from build123d import *

# Parameters (mm, degrees)
TRAY_BLOCK_DEPTH              = 24.4
LOWER_FRONT_FACET_DEPTH       = 74.975401317
LOWER_FRONT_FACET_DEPTH_BACK  = 74.975401317
LOWER_SIDE_FACET_L_DEPTH      = 74.975401317
LOWER_SIDE_FACET_L_DEPTH_BACK = 74.975401317
LOWER_SIDE_FACET_R_DEPTH      = 74.975401317
LOWER_SIDE_FACET_R_DEPTH_BACK = 74.975401317
SHELL_T                       = -2.4
SEAM_REBATE_DEPTH             = 4.3
SKETCH6_R                     = 2.5
BOARD_PILLARS_DEPTH           = 24.9
SKETCH7_R                     = 0.8
BOARD_PILOTS_DEPTH            = 8.5
SKETCH8_W                     = 40
SKETCH8_H                     = 21
CABLE_WINDOW_DEPTH            = 3.9
SKETCH9_R                     = 4
FLANGE_BOSSES_DEPTH           = 6.2
SKETCH10_R                    = 2
FLANGE_INSERT_HOLES_DEPTH     = 7
SKETCH11_R                    = 1.7
SEAM_SCREW_HOLE_L_DEPTH       = 3.9
SKETCH12_R                    = 1.7
SEAM_SCREW_HOLE_R_DEPTH       = 3.9
SKETCH13_W                    = 12
SKETCH13_H                    = 7
BUNDLE_TIE_ANCHOR_DEPTH       = 5
SKETCH14_W                    = 4
SKETCH14_H                    = 2
BUNDLE_TIE_SLOT_DEPTH         = 14
SKETCH15_R                    = 1.5
DRAIN_HOLE_DEPTH              = 3.9


with BuildPart() as part:
    # Sketch1 → Tray Block (new body)
    with BuildSketch(Plane(origin=(0, -28.4, 0), x_dir=(1, 0, 0), z_dir=(0, 1, 0))):
        Polygon((-48.4, -11.9), (48.4, -11.9), (48.4, 42.2), (42.4, 48.2), (-42.4, 48.2), (-48.4, 42.2), align=None)
    extrude(amount=TRAY_BLOCK_DEPTH)

    # Sketch2 → Lower Front Facet (cut, two sides: drawn at the far end of the back side and taken through both)
    with BuildSketch(Plane(origin=(0, 0, 0), x_dir=(0, 0, -1), z_dir=(1, 0, 0)).offset(-LOWER_FRONT_FACET_DEPTH_BACK)):
        Polygon((49.64, -6.32), (53.2, -6.32), (53.2, -32.08), (39.56, -32.08), align=None)
    extrude(amount=LOWER_FRONT_FACET_DEPTH + LOWER_FRONT_FACET_DEPTH_BACK, mode=Mode.SUBTRACT)

    # Sketch3 → Lower Side Facet L (cut, two sides: drawn at the far end of the back side and taken through both)
    with BuildSketch(Plane.XY.offset(-LOWER_SIDE_FACET_L_DEPTH_BACK)):
        Polygon((-49.4, -21.4), (-49.4, -29.4), (-41.4, -29.4), align=None)
    extrude(amount=LOWER_SIDE_FACET_L_DEPTH + LOWER_SIDE_FACET_L_DEPTH_BACK, mode=Mode.SUBTRACT)

    # Sketch4 → Lower Side Facet R (cut, two sides: drawn at the far end of the back side and taken through both)
    with BuildSketch(Plane.XY.offset(-LOWER_SIDE_FACET_R_DEPTH_BACK)):
        Polygon((49.4, -21.4), (49.4, -29.4), (41.4, -29.4), align=None)
    extrude(amount=LOWER_SIDE_FACET_R_DEPTH + LOWER_SIDE_FACET_R_DEPTH_BACK, mode=Mode.SUBTRACT)

    # Shell
    shell_openings = [part.faces().sort_by_distance(p)[0] for p in [
        (0, -4, -17.975344882),
    ]]
    offset(amount=SHELL_T, openings=shell_openings, kind=Kind.INTERSECTION)

    # Sketch5 → Seam Rebate (cut)
    with BuildSketch(Plane(origin=(0, -7.3, 0), x_dir=(1, 0, 0), z_dir=(0, 1, 0))):
        Polygon((-46.3, -9.8), (46.3, -9.8), (46.3, 41.330151519), (41.530151519, 46.1), (-41.530151519, 46.1), (-46.3, 41.330151519), align=None)
    extrude(amount=SEAM_REBATE_DEPTH, mode=Mode.SUBTRACT)

    # Sketch6 → Board Pillars (add)
    with BuildSketch(Plane(origin=(0, -26.5, 0), x_dir=(1, 0, 0), z_dir=(0, 1, 0))):
        with Locations(Location((-11.3, 11.8, 0), (0, 0, 270))):
            Circle(SKETCH6_R)
        with Locations(Location((-11.3, 34.9, 0), (0, 0, 270))):
            Circle(SKETCH6_R)
        with Locations(Location((11.3, 11.8, 0), (0, 0, 270))):
            Circle(SKETCH6_R)
        with Locations(Location((11.3, 34.9, 0), (0, 0, 270))):
            Circle(SKETCH6_R)
    extrude(amount=BOARD_PILLARS_DEPTH)

    # Sketch7 → Board Pilots (cut)
    with BuildSketch(Plane(origin=(0, -9.6, 0), x_dir=(1, 0, 0), z_dir=(0, 1, 0))):
        with Locations(Location((-11.3, 11.8, 0), (0, 0, 270))):
            Circle(SKETCH7_R)
        with Locations(Location((-11.3, 34.9, 0), (0, 0, 270))):
            Circle(SKETCH7_R)
        with Locations(Location((11.3, 11.8, 0), (0, 0, 270))):
            Circle(SKETCH7_R)
        with Locations(Location((11.3, 34.9, 0), (0, 0, 270))):
            Circle(SKETCH7_R)
    extrude(amount=BOARD_PILOTS_DEPTH, mode=Mode.SUBTRACT)

    # Sketch8 → Cable Window (cut)
    with BuildSketch(Plane.XY.offset(9)):
        with Locations((0, -13.5)):
            Rectangle(SKETCH8_W, SKETCH8_H)
    extrude(amount=CABLE_WINDOW_DEPTH, mode=Mode.SUBTRACT)

    # Sketch9 → Flange Bosses (add)
    with BuildSketch(Plane.XY.offset(3.5)):
        with Locations(Location((-32, -20, 0), (0, 0, 180))):
            Circle(SKETCH9_R)
        with Locations(Location((32, -20, 0), (0, 0, 180))):
            Circle(SKETCH9_R)
    extrude(amount=FLANGE_BOSSES_DEPTH)

    # Sketch10 → Flange Insert Holes (cut)
    with BuildSketch(Plane.XY.offset(5.4)):
        with Locations(Location((-32, -20, 0), (0, 0, 180))):
            Circle(SKETCH10_R)
        with Locations(Location((32, -20, 0), (0, 0, 180))):
            Circle(SKETCH10_R)
    extrude(amount=FLANGE_INSERT_HOLES_DEPTH, mode=Mode.SUBTRACT)

    # Sketch11 → Seam Screw Hole L (cut)
    with BuildSketch(Plane(origin=(-49.4, 0, 0), x_dir=(0, 0, -1), z_dir=(1, 0, 0))):
        with Locations(Location((34, -8, 0), (0, 0, 155.684260829))):
            Circle(SKETCH11_R)
    extrude(amount=SEAM_SCREW_HOLE_L_DEPTH, mode=Mode.SUBTRACT)

    # Sketch12 → Seam Screw Hole R (cut)
    with BuildSketch(Plane(origin=(45.5, 0, 0), x_dir=(0, 0, -1), z_dir=(1, 0, 0))):
        with Locations(Location((34, -8, 0), (0, 0, 155.684260829))):
            Circle(SKETCH12_R)
    extrude(amount=SEAM_SCREW_HOLE_R_DEPTH, mode=Mode.SUBTRACT)

    # Sketch13 → Bundle Tie Anchor (add)
    with BuildSketch(Plane(origin=(0, -26.5, 0), x_dir=(1, 0, 0), z_dir=(0, 1, 0))):
        with Locations((0, -5.5)):
            Rectangle(SKETCH13_W, SKETCH13_H)
    extrude(amount=BUNDLE_TIE_ANCHOR_DEPTH)

    # Sketch14 → Bundle Tie Slot (cut)
    with BuildSketch(Plane(origin=(-7, 0, 0), x_dir=(0, 0, -1), z_dir=(1, 0, 0))):
        with Locations((-5.5, -25)):
            Rectangle(SKETCH14_W, SKETCH14_H)
    extrude(amount=BUNDLE_TIE_SLOT_DEPTH, mode=Mode.SUBTRACT)

    # Sketch15 → Drain Hole (cut)
    with BuildSketch(Plane(origin=(0, -29.4, 0), x_dir=(1, 0, 0), z_dir=(0, 1, 0))):
        with Locations(Location((0, 34, 0), (0, 0, 270))):
            Circle(SKETCH15_R)
    extrude(amount=DRAIN_HOLE_DEPTH, mode=Mode.SUBTRACT)


solid = part.part
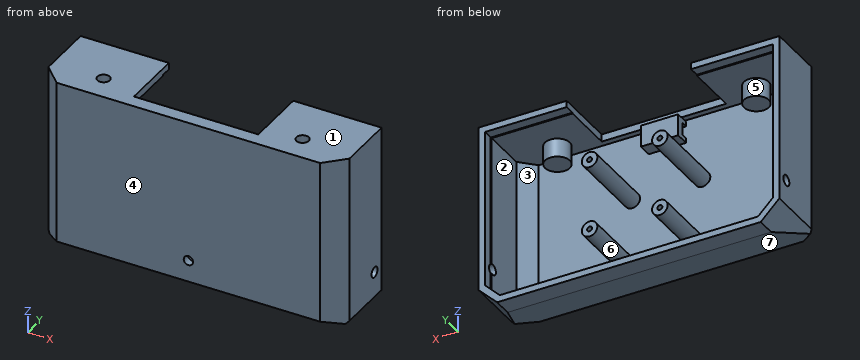
The model under review builds one solid part; all positions refer to its coordinate system, in mm. Face numbers are marked on the shaded views. A direction names the side the tool comes from. Coordinates: 2 decimals unless noted, no trailing zeros. Loops run counter-clockwise (first coordinate to the right, second up) from the corner with the lowest first, then second, coordinate; pieces in that order, holes last. Notation, with made-up numbers: M 2,87 L 15,87 A19 cw 15,91 Z; hole C -16.5,-16 d11. An arc over 180 degrees is marked long. Put each result on its own line as item: value. Start each with the question number.
Q1. Add section A-A (y = -8.25). Count the separate pieces of the cut face and the enclosed holes in it, and give its area (3 significant figures).
Q2. The part is to be moulded in two halves that separate along Z. For the marked faces 1, 2, 3 and 4, say which applies: +Z half, -Z half, draft (parallel to the pull), parting line (faces both ways), or undercut.
Q3. For the marked faces 5, 6 and 7, list the 3-axis set-ups (+Z, -Z, +X, -X, +Y, -Y) from which the entire face can be reached by the end or side of a thin tool; tool diameter is ignored.
Q4. Clearance check with flat-ended pins moving along their axes: pin 1 (2 mm diameter, centred on x = -31.5, y = -20, fed in from +Z); pin 2 (8 mm diameter, centred on x = 31.5, z = -18.5, fed in from +Y); pin 3 (1.3 mm diameter, centred on y = -24, z = 6.5, fed in from +X). State where each tip first meets the part, or that it passes through.
Q5. Add section D-D (x = -2.5). Write out the cut boundary in (y, z), and give its area (3 significant figures).
Q6. Add section C-C (z = -27). Write out the cut boundary in (x, y).
Q7. Add section B-B (x = -32). Write out the cut boundary in (y, z), and give its area (3 significant figures).
Q8. Wall thickness on line 1 (X direction, y = -20, z = 8); line 2 (Y direction, x = -32, z = 7.75); line 3 (X direction, y = -5.5, z = -11.8): over which ranges is each line inside the solid? List them lowest first.
Answers:
1. separate pieces: 7
1. enclosed holes: 4
1. area: 674 mm^2
2. face 1: +Z half
2. face 2: undercut
2. face 3: undercut
2. face 4: draft
3. face 5: none
3. face 6: +Y
3. face 7: -Z, +X, -X, -Y
4. pin 1: stops at z = 5.4
4. pin 2: stops at y = -26
4. pin 3: stops at x = 47.45
5. outline: M -28.4,-41 L -10,-48.2 L -4,-48.2 L -4,-46.1 L -7.3,-46.1 L -7.3,-45.8 L -9.55,-45.8 L -26,-39.36 L -26,2 L -21.5,2 L -21.5,9 L -26,9 L -26,9.5 L -24,9.5 L -24,11.9 L -28.4,11.9 Z; hole M -26,3.5 L -24,3.5 L -24,7.5 L -26,7.5 Z
5. area: 211 mm^2
6. outline: M -48.4,-22.4 L -42.4,-28.4 L 42.4,-28.4 L 48.4,-22.4 L 48.4,-4 L 46.3,-4 L 46.3,-7.3 L 46,-7.3 L 46,-21.41 L 41.41,-26 L -41.41,-26 L -46,-21.41 L -46,-7.3 L -46.3,-7.3 L -46.3,-4 L -48.4,-4 Z
7. outline: M -28.4,-41 L -10,-48.2 L -4,-48.2 L -4,-46.1 L -7.3,-46.1 L -7.3,-45.8 L -9.55,-45.8 L -26,-39.36 L -26,9.5 L -24,9.5 L -24,3.5 L -16,3.5 L -16,9.5 L -7.3,9.5 L -7.3,9.8 L -4,9.8 L -4,11.9 L -18,11.9 L -18,5.4 L -22,5.4 L -22,11.9 L -28.4,11.9 Z
7. area: 257 mm^2
8. line 1: x = -48.4 to -46, -36 to -34, -30 to -28, 28 to 30, 34 to 36, 46 to 48.4
8. line 2: y = -28.4 to -26, -24 to -22, -18 to -16
8. line 3: x = -48.4 to -46.3, -13.8 to -12.1, -10.5 to -8.8, 8.8 to 10.5, 12.1 to 13.8, 46.3 to 48.4
